```python
from build123d import *

# Parameters (mm, degrees)
ESBO_O1_W                 = 204
ESBO_O1_H                 = 104
RESSALTO_EXTRUS_O1_DEPTH  = 52
CORTE_EXTRUS_O1_DEPTH     = 50
FILETE1_R                 = 5
CORTE_EXTRUS_O2_DEPTH     = 40
CORTE_EXTRUS_O5_DEPTH     = 3
CORTE_EXTRUS_O6_START     = -53
ESBO_O8_R                 = 2.5
CORTE_EXTRUS_O6_DEPTH     = 54
ESPELHAR2_COPY_1_DEPTH    = 40
ESPELHAR2_COPY_2_DEPTH    = 3
ESPELHAR2_START           = -53
ESPELHAR2_COPY_3_SKETCH_R = 2.5
ESPELHAR2_COPY_3_DEPTH    = 54


with BuildPart() as part:
    # Esboço1 → Ressalto-extrusão1 (new body)
    with BuildSketch(Plane.XY):
        Rectangle(ESBO_O1_W, ESBO_O1_H)
    extrude(amount=-RESSALTO_EXTRUS_O1_DEPTH)

    # Esboço2 → Corte-extrusão1 (cut)
    with BuildSketch(Plane.XY):
        with BuildLine():
            Line((-87, 50), (87, 50))
            Line((87, 50), (87, 42))
            ThreePointArc((87, 42), (88.464466094, 38.464466094), (92, 37))
            Line((92, 37), (100, 37))
            Line((100, 37), (100, -37))
            Line((100, -37), (92, -37))
            ThreePointArc((92, -37), (88.464466094, -38.464466094), (87, -42))
            Line((87, -42), (87, -50))
            Line((87, -50), (-87, -50))
            Line((-87, -50), (-87, -42))
            ThreePointArc((-87, -42), (-88.464466094, -38.464466094), (-92, -37))
            Line((-92, -37), (-100, -37))
            Line((-100, -37), (-100, 37))
            Line((-100, 37), (-92, 37))
            ThreePointArc((-92, 37), (-88.464466094, 38.464466094), (-87, 42))
            Line((-87, 42), (-87, 50))
        make_face()
    extrude(amount=-CORTE_EXTRUS_O1_DEPTH, mode=Mode.SUBTRACT)

    # Filete1
    filete1_edges = [part.edges().sort_by_distance(p)[0] for p in [
        (102, -52, -26),
        (-102, -52, -26),
        (-102, 52, -26),
        (102, 52, -26),
    ]]
    fillet(filete1_edges, radius=FILETE1_R)

    # Esboço4 → Corte-extrusão2 (cut)
    with BuildSketch(Plane(origin=(0, 0, -52), x_dir=(-1, 0, 0), z_dir=(0, 0, -1))):
        with BuildLine():
            Line((-97, 50), (-90, 50))
            Line((-90, 50), (-90, 43))
            ThreePointArc((-90, 43), (-90.878679656, 40.878679656), (-93, 40))
            Line((-93, 40), (-100, 40))
            Line((-100, 40), (-100, 47))
            ThreePointArc((-100, 47), (-99.121320344, 49.121320344), (-97, 50))
        make_face()
    corte_extrus_o2 = extrude(amount=-CORTE_EXTRUS_O2_DEPTH, mode=Mode.SUBTRACT)

    # Esboço7 → Corte-extrusão5 (cut)
    with BuildSketch(Plane.XY):
        with BuildLine():
            Line((-102, 40), (-93, 40))
            ThreePointArc((-93, 40), (-90.878679656, 40.878679656), (-90, 43))
            Line((-90, 43), (-90, 52))
            Line((-90, 52), (-97, 52))
            ThreePointArc((-97, 52), (-100.535533906, 50.535533906), (-102, 47))
            Line((-102, 47), (-102, 40))
        make_face()
    corte_extrus_o5 = extrude(amount=-CORTE_EXTRUS_O5_DEPTH, mode=Mode.SUBTRACT)

    # Esboço8 → Corte-extrusão6 (cut)
    with BuildSketch(Plane.XY.offset(CORTE_EXTRUS_O6_START)):
        with Locations((-94.5, 45)):
            Circle(ESBO_O8_R)
    corte_extrus_o6 = extrude(amount=CORTE_EXTRUS_O6_DEPTH, mode=Mode.SUBTRACT)

    # Espelhar1: Corte-extrusão2, Corte-extrusão5, Corte-extrusão6 across plane
    add(corte_extrus_o2.mirror(Plane(origin=(0, 0, 0), x_dir=(0, 0, 1), z_dir=(1, 0, 0))), mode=Mode.SUBTRACT)
    add(corte_extrus_o5.mirror(Plane(origin=(0, 0, 0), x_dir=(0, 0, 1), z_dir=(1, 0, 0))), mode=Mode.SUBTRACT)
    add(corte_extrus_o6.mirror(Plane(origin=(0, 0, 0), x_dir=(0, 0, 1), z_dir=(1, 0, 0))), mode=Mode.SUBTRACT)

    # Espelhar2: Corte-extrusão2, Corte-extrusão5, Corte-extrusão6 across plane
    add(corte_extrus_o2.mirror(Plane.ZX), mode=Mode.SUBTRACT)
    add(corte_extrus_o5.mirror(Plane.ZX), mode=Mode.SUBTRACT)
    add(corte_extrus_o6.mirror(Plane.ZX), mode=Mode.SUBTRACT)

    # Espelhar2 copy 1 sketch → Espelhar2 copy 1 (cut)
    with BuildSketch(Plane(origin=(0, 0, -52), x_dir=(1, 0, 0), z_dir=(0, 0, -1))):
        with BuildLine():
            Line((-97, 50), (-90, 50))
            Line((-90, 50), (-90, 43))
            ThreePointArc((-90, 43), (-90.878679656, 40.878679656), (-93, 40))
            Line((-93, 40), (-100, 40))
            Line((-100, 40), (-100, 47))
            ThreePointArc((-100, 47), (-99.121320344, 49.121320344), (-97, 50))
        make_face()
    extrude(amount=-ESPELHAR2_COPY_1_DEPTH, mode=Mode.SUBTRACT)

    # Espelhar2 copy 2 sketch → Espelhar2 copy 2 (cut)
    with BuildSketch(Plane(origin=(0, 0, 0), x_dir=(-1, 0, 0), z_dir=(0, 0, 1))):
        with BuildLine():
            Line((-102, 40), (-93, 40))
            ThreePointArc((-93, 40), (-90.878679656, 40.878679656), (-90, 43))
            Line((-90, 43), (-90, 52))
            Line((-90, 52), (-97, 52))
            ThreePointArc((-97, 52), (-100.535533906, 50.535533906), (-102, 47))
            Line((-102, 47), (-102, 40))
        make_face()
    extrude(amount=-ESPELHAR2_COPY_2_DEPTH, mode=Mode.SUBTRACT)

    # Espelhar2 copy 3 sketch → Espelhar2 copy 3 (cut)
    with BuildSketch(Plane(origin=(0, 0, 0), x_dir=(-1, 0, 0), z_dir=(0, 0, 1)).offset(ESPELHAR2_START)):
        with Locations((-94.5, 45)):
            Circle(ESPELHAR2_COPY_3_SKETCH_R)
    extrude(amount=ESPELHAR2_COPY_3_DEPTH, mode=Mode.SUBTRACT)


solid = part.part
```
For this review, take the finished solid that the model builds, in its own axes (mm). A direction names the side the tool comes from. Give positions to 0.01 mm unless a question says otherwise; leave off trailing zeros. Write each loop counter-clockwise with the first axis right and the second up, starting at its lowest first coordinate (ties: lowest second). Pieces come first, ordered by that corner, then holes. Notation, with made-up numbers: M 53.25,-5.5 L 61.25,-5.5 A15 cw 61.25,1.5 Z; hole C 42.5,83 d8. An arc over 180 degrees is marked long. Answer as a JSON object with one key per item and string values. Group by question number.
Item 1: Draft analysis for pull direction X (two halves, no side actions). For faces 5 (the flat face through (-1, 52, -26)), 6 (the flat face through (90, -47, -32)), 7 (the cylindrical face through (-101, -50, -28)), state which applies: +X half, -X half, draft (parallel to the pull), parting line (faces both ways), or undercut.
Item 2: Tool access review of faces 1 (the flat face through (-1, 50, -25)), 2 (the flat face through (-97, 46, -3)), 3 (the flat face through (97.2, -45.1, -12)), 4 (the flat face through (97, 46, -3)): name each direction out of +Z, -Z, +X, -X, +Y, -Y from which nothing blocks a thin tool from reaching the whole face with its end or side.
Item 3: For pin 1 Ø1.5 at (x, z) = (-96.5, -2) entering from +Y; pin 2 Ø5 at (x, y) = (-95.5, 43.5) entering from -Z; pin 3 Ø2 at (x, y) = (75, 12.5) entering from +Z, all flat-tipped, find the tip position at first contact; note any pin that passes through.
Item 4: Consider section A-A on y = -45. Write out the cut boundary in (x, z), plus the area to 3 significant figures.
Item 5: For probe 1 along X at (y, z) = (-12, -40.5); probe 2 along Y at (x, z) = (-58.5, -10); probe 3 along Y at (x, z) = (94.5, -7.5), list the stretches that pass through material, from the lowest coordinate up. Write a range as [from, to].
Item 6: Consider section C-C on z = -26. Count the separate pieces of the cut face and the enclosed holes in it, plus the area to 3 significant figures.
Item 7: Consider section B-B on x = -83.5. Write out the cut boundary in (y, z).
Check result:
{
 "1": {"face 5": "draft", "face 6": "undercut", "face 7": "-X half"},
 "2": {"face 1": "+Z", "face 2": "+Z, -X, +Y", "face 3": "-Z", "face 4": "+Z, +X, +Y"},
 "3": {"pin 1": "stops at y = 40", "pin 2": "stops at z = -12", "pin 3": "stops at z = -50"},
 "4": {"outline": "M -102,-52 L -100,-52 L -100,-12 L -97,-12 L -97,-3 L -102,-3 Z; M -92,-12 L -90,-12 L -90,-52 L 90,-52 L 90,-12 L 92,-12 L 92,-3 L 90,-3 L 90,0 L 87,0 L 87,-50 L -87,-50 L -87,0 L -90,0 L -90,-3 L -92,-3 Z; M 97,-12 L 100,-12 L 100,-52 L 102,-52 L 102,-3 L 97,-3 Z", "area": "946 mm^2"},
 "5": {"probe 1": "x = [-102, -100], [100, 102]", "probe 2": "y = [-52, -50], [50, 52]", "probe 3": "y = [-52, -47.5], [-42.5, -37], [37, 42.5], [47.5, 52]"},
 "6": {"separate pieces": "1", "enclosed holes": "5", "area": "1,460 mm^2"},
 "7": {"outline": "M -52,-52 L 52,-52 L 52,0 L 50,0 L 50,-50 L -50,-50 L -50,0 L -52,0 Z"}
}
